Autodesk Fusion 360 part; units mm, degrees
sketch "Sketch1" plane through (0, 0, 0) normal (0, 1, 0) x (1, 0, 0)
  line L0 (0, 0) -> (35, 0)
  line L1 (35, 0) -> (35, -9)
  line L2 (35, -9) -> (0, -9)
  line L3 (0, -9) -> (0, 0)
  dimension "d1" = 35
  dimension "d2" = 9
extrude "Extrude1" add sketch "Sketch1" along normal blind 0.5
extrude "Extrude2" add 1 faces at (11.6667, 0.5, 3) along direction (0, 1, 0) blind 0.2
sketch "Sketch2" plane through (0, 0.7, 0) normal (0, 1, 0) x (-1, 0, 0)
  line L0 (0, 9) -> (-35, 9)
  line L1 (-35, 9) -> (-35, 0)
  line L2 (-35, 0) -> (0, 0)
  line L3 (0, 0) -> (0, 9)
  line L4 (0, 0) -> (-2, 0)
  line L5 (-2, 0) -> (-2, 9)
  line L6 (-2, 9) -> (0, 9)
  line L7 (0, 9) -> (0, 0)
  dimension "d7" = 2
extrude "Extrude3" add sketch "Sketch2" along normal blind 8.3 contours L0 L2 L3 L4 L5 L6 L7
sketch "Sketch3" plane through (2, 0, 0) normal (1, 0, 0) x (0, 0, -1)
  line L0 (-9, 0.7) -> (0, 0.7)
  line L1 (0, 0.7) -> (0, 9)
  line L2 (0, 9) -> (-9, 9)
  line L3 (-9, 9) -> (-9, 0.7)
  line L4 (-9, 9) -> (-4.5, 9)
  line L5 (-4.5, 9) -> (-4.5, 4.85)
  line L6 (-4.5, 4.85) -> (-9, 4.85)
  line L7 (-9, 4.85) -> (-9, 9)
  line L8 (-4.5, 9) -> (0, 9)
  line L9 (0, 9) -> (0, 4.85)
  line L10 (0, 4.85) -> (-4.5, 4.85)
  line L11 (-4.5, 4.85) -> (-4.5, 9)
  line L12 (-9, 4.85) -> (-4.5, 4.85)
  line L13 (-4.5, 4.85) -> (-4.5, 0.7)
  line L14 (-4.5, 0.7) -> (-9, 0.7)
  line L15 (-9, 0.7) -> (-9, 4.85)
  line L16 (-4.5, 4.85) -> (0, 4.85)
  line L17 (0, 4.85) -> (0, 0.7)
  line L18 (0, 0.7) -> (-4.5, 0.7)
  line L19 (-4.5, 0.7) -> (-4.5, 4.85)
  circle A0 centre (-6.75, 6.925) radius 0.75
  circle A1 centre (-2.25, 6.925) radius 0.75
  circle A2 centre (-6.75, 2.775) radius 0.75
  circle A3 centre (-2.25, 2.775) radius 0.75
  dimension "d10" = 4.5
  dimension "d11" = 4.15
  dimension "d12" = 1.5
  dimension "d13" = 1.5
  dimension "d14" = 1.5
  dimension "d15" = 1.5
extrude "Extrude4" cut sketch "Sketch3" against normal up to surface (2 mm away) contours A0 | A1 | A2 | A3
sketch "Sketch4" plane through (0, 0.7, 0) normal (0, 1, 0) x (-1, 0, 0)
  line L0 (-2, 0) -> (-2, 9)
  line L1 (-2, 9) -> (-35, 9)
  line L2 (-35, 9) -> (-35, 0)
  line L3 (-35, 0) -> (-2, 0)
  line L4 (-35, 9) -> (-33, 9)
  line L5 (-33, 9) -> (-33, 0)
  line L6 (-33, 0) -> (-35, 0)
  line L7 (-35, 0) -> (-35, 9)
  dimension "d18" = 2
extrude "Extrude5" add sketch "Sketch4" along normal up to surface (8.3 mm away) contours L1 L2 L3 L4 L5 L6 L7
sketch "Sketch5" plane through (33, 0, 0) normal (-1, 0, 0) x (0, 0, 1)
  line L0 (9, 9) -> (0, 9)
  line L1 (0, 9) -> (0, 0.7)
  line L2 (0, 0.7) -> (9, 0.7)
  line L3 (9, 0.7) -> (9, 9)
  line L4 (6, 3.35) -> (3, 3.35)
  line L5 (3, 3.35) -> (3, 6.35)
  line L6 (3, 6.35) -> (6, 6.35)
  line L7 (6, 6.35) -> (6, 3.35)
  line L8 (6, 3.35) -> (3, 6.35) construction
  line L9 (3, 3.35) -> (6, 6.35) construction
  point P0 (4.5, 4.85)
  point P1 (4.5, 4.85)
  dimension "d21" = 3
  dimension "d22" = 3
extrude "Extrude6" cut sketch "Sketch5" against normal up to surface (2 mm away) contours L4 L5 L6 L7
delete_face "DeleteFace1" 1 faces at (0.6667, 6.8503, 1.5037)
delete_face "DeleteFace2" 1 faces at (0.6667, 6.8503, 6.0037)
delete_face "DeleteFace3" 1 faces at (0.6667, 2.7003, 6.0037)
delete_face "DeleteFace4" 1 faces at (0.6667, 2.7003, 1.5037)
delete_face "DeleteFace5" 1 faces at (33.6667, 4.35, 3)
sketch "Sketch6" plane through (35, 0, 0) normal (1, 0, 0) x (0, 0, -1)
  line L0 (0, 0) -> (0, 9)
  line L1 (0, 9) -> (-9, 9)
  line L2 (-9, 9) -> (-9, 0)
  line L3 (-9, 0) -> (0, 0)
  line L4 (-9, 9) -> (-7.5, 9)
  line L5 (-7.5, 9) -> (-7.5, 7.5)
  line L6 (-7.5, 7.5) -> (-9, 7.5)
  line L7 (-9, 7.5) -> (-9, 9)
  line L8 (0, 9) -> (-1.5, 9)
  line L9 (-1.5, 9) -> (-1.5, 7.5)
  line L10 (-1.5, 7.5) -> (0, 7.5)
  line L11 (0, 7.5) -> (0, 9)
  line L12 (-9, 0) -> (-7.5, 0)
  line L13 (-7.5, 0) -> (-7.5, 1.5)
  line L14 (-7.5, 1.5) -> (-9, 1.5)
  line L15 (-9, 1.5) -> (-9, 0)
  line L16 (0, 0) -> (-1.5, 0)
  line L17 (-1.5, 0) -> (-1.5, 1.5)
  line L18 (-1.5, 1.5) -> (0, 1.5)
  line L19 (0, 1.5) -> (0, 0)
  line L20 (-7.5, 7.5) -> (-1.5, 7.5)
  line L21 (-1.5, 7.5) -> (-1.5, 1.5)
  line L22 (-1.5, 1.5) -> (-7.5, 1.5)
  line L23 (-7.5, 1.5) -> (-7.5, 7.5)
  dimension "d25" = 1.5
  dimension "d26" = 1.5
  dimension "d27" = 1.5
  dimension "d28" = 1.5
  dimension "d29" = 1.5
  dimension "d30" = 1.5
  dimension "d31" = 1.5
  dimension "d32" = 1.5
extrude "Extrude7" cut sketch "Sketch6" against normal up to surface (2 mm away) contours L20 L21 L22 L23
sketch "Sketch7" plane through (0, 0, 0) normal (-1, 0, 0) x (0, 0, 1)
  line L0 (0, 0) -> (9, 0)
  line L1 (9, 0) -> (9, 9)
  line L2 (9, 9) -> (0, 9)
  line L3 (0, 9) -> (0, 0)
  line L4 (0, 9) -> (1.5, 9)
  line L5 (1.5, 9) -> (1.5, 7.5)
  line L6 (1.5, 7.5) -> (0, 7.5)
  line L7 (0, 7.5) -> (0, 9)
  line L8 (9, 9) -> (7.5, 9)
  line L9 (7.5, 9) -> (7.5, 7.5)
  line L10 (7.5, 7.5) -> (9, 7.5)
  line L11 (9, 7.5) -> (9, 9)
  line L12 (0, 0) -> (1.5, 0)
  line L13 (1.5, 0) -> (1.5, 1.5)
  line L14 (1.5, 1.5) -> (0, 1.5)
  line L15 (0, 1.5) -> (0, 0)
  line L16 (9, 0) -> (7.5, 0)
  line L17 (7.5, 0) -> (7.5, 1.5)
  line L18 (7.5, 1.5) -> (9, 1.5)
  line L19 (9, 1.5) -> (9, 0)
  line L20 (1.5, 7.5) -> (7.5, 7.5)
  line L21 (7.5, 7.5) -> (7.5, 1.5)
  line L22 (7.5, 1.5) -> (1.5, 1.5)
  line L23 (1.5, 1.5) -> (1.5, 7.5)
  dimension "d35" = 1.5
  dimension "d36" = 1.5
  dimension "d37" = 1.5
  dimension "d38" = 1.5
  dimension "d39" = 1.5
  dimension "d40" = 1.5
  dimension "d41" = 1.5
  dimension "d42" = 1.5
extrude "Extrude8" cut sketch "Sketch7" against normal up to surface (2 mm away) contours L20 L21 L22 L23
Part model, mm, in its own coordinate system. A direction names the side the tool comes from. Coordinates: 2 decimals unless noted, no trailing zeros. Order: outer loops, then holes, each group sorted by start corner. A loop starts at its lowest first (then second) coordinate and runs counter-clockwise, first axis right, second up. Notation, with made-up numbers: (46, -39) -> (104, -39) arc R9 cw to (104, -29) -> close; hole circle Ø3 at (89.25, 40.5). An arc over 180 degrees is marked (long way). Put each result on its own line as item: value. Start each with the question number.
(1) Pin check, flat tip, straight feed: pin 1 Ø1.5 at (x, z) = (12, 5.5) entering from +Y. Stop position of the tip, or through.
(2) Band-saw the part on B-B (z = 6). Give the cut face in (x, y), then the cut area to 3 significant figures.
(3) Mould opens along Y. For faces 1 (the face through (0, 4, 1)), 2 (the face through (17, 0.7, 4)), 3 (the face through (1, 7.5, 4)) say: pulls with the +Y half, pulls with the -Y half, needs draft (parallel to the pull), parting line crosses it, or undercut.
(4) Band-saw the part on A-A (y = 1). Give the cut face in (x, z).
(5) Band-saw the part on C-C (y = 3). Give the cut face in (x, z).
(6) Which spindle directions (+Z, -Z, +X, -X, +Y, -Y) get a long thin tool onto all of the face, cutting with end or side? Do faces 4 (the face through (33, 8, 5)), 5 (the face through (34, 4, 7.5)), 6 (the face through (35, 1, 5)). Say none if no direction does.
(7) Band-saw the part on D-D (z = 8). Give the cut face in (x, y).
(8) Probe line 1 along X through (y, z) = (8.5, 6.25); line 2 along Y through (x, z) = (31.5, 2.5). List the from-to ranges inside material, lowest first. Write a range as [from, to].
Determined:
1. pin 1: stops at y = 0.7
2. outline: (0, 0) -> (35, 0) -> (35, 1.5) -> (33, 1.5) -> (33, 0.7) -> (2, 0.7) -> (2, 1.5) -> (0, 1.5) -> close; (0, 7.5) -> (2, 7.5) -> (2, 9) -> (0, 9) -> close; (33, 7.5) -> (35, 7.5) -> (35, 9) -> (33, 9) -> close
2. area: 33.7 mm²
3. face 1: needs draft
3. face 2: pulls with the +Y half
3. face 3: undercut
4. outline: (0, 0) -> (2, 0) -> (2, 9) -> (0, 9) -> close; (33, 0) -> (35, 0) -> (35, 9) -> (33, 9) -> close
5. outline: (0, 0) -> (2, 0) -> (2, 1.5) -> (0, 1.5) -> close; (0, 7.5) -> (2, 7.5) -> (2, 9) -> (0, 9) -> close; (33, 0) -> (35, 0) -> (35, 1.5) -> (33, 1.5) -> close; (33, 7.5) -> (35, 7.5) -> (35, 9) -> (33, 9) -> close
6. face 4: +Z, -Z, +Y
6. face 5: +X, -X
6. face 6: +Z, -Z, +X, +Y, -Y
7. outline: (0, 0) -> (35, 0) -> (35, 9) -> (33, 9) -> (33, 0.7) -> (2, 0.7) -> (2, 9) -> (0, 9) -> close
8. line 1: x = [0, 2], [33, 35]
8. line 2: y = [0, 0.7]
